Autodesk Inventor part; units mm, degrees
ref_plane "YZ Plane" through (0, 0, 0) normal (1, 0, 0) x (0, 1, 0)
ref_plane "XZ Plane" through (0, 0, 0) normal (0, 1, 0) x (-1, 0, 0)
ref_plane "XY Plane" through (0, 0, 0) normal (0, 0, 1) x (1, 0, 0)
sketch "Sketch1" plane through (0, 0, 0) normal (0, 0, 1) x (1, 0, 0)
  line L0 (-2.75, 1.59) -> (0, 3.18)
  line L1 (0, -3.18) -> (-2.75, -1.59)
  line L2 (-2.75, 1.59) -> (-2.75, -1.59)
  line L3 (2.75, 1.59) -> (0, 3.18)
  line L4 (0, -3.18) -> (2.75, -1.59)
  line L5 (2.75, 1.59) -> (2.75, -1.59)
  point P0 (0, 0)
extrude "Extrusion1" add sketch "Sketch1" along normal blind 6
sketch "Sketch2" plane through (0, 0, 6) normal (0, 0, 1) x (1, 0, 0)
  circle A0 centre (0, 0) radius 1.5
  dimension "d20" = 3
hole "Hole1" at (0, 0, 6) direction (0, 0, -1) diameter 2.459 depth 8.8 tip angle 118
fillet "Fillet1" radius 0.1 6 edges at (0, 3.18, 3) (2.75, 1.59, 3) (-2.75, 1.59, 3) (2.75, -1.59, 3) (0, -3.18, 3) (-2.75, -1.59, 3)
sketch "Sketch4" plane through (0, 0, 0) normal (0, 0, -1) x (-1, 0, 0)
  circle A0 centre (0, 0) radius 1.5
  dimension "d29" = 3
extrude "Extrusion2" add sketch "Sketch4" along normal blind 6.4
thread "Thread1"
fillet "Fillet2" radius 0.2 1 edges at (1.5, 0, -6.4)
properties part number "spacer 3cm" material "Steel, Mild"
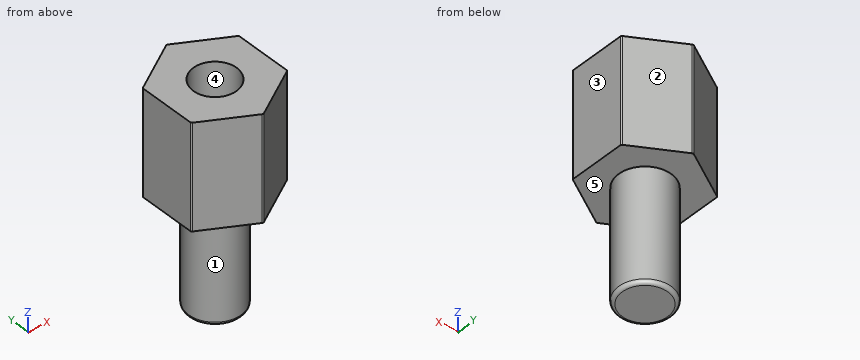
Here's how the part is built. I have some questions about the finished solid (model axes, mm). Face numbers are marked on the shaded views. A direction names the side the tool comes from. Coordinates: 2 decimals unless noted, no trailing zeros. Write each loop counter-clockwise with the first axis right and the second up, starting at its lowest first coordinate (ties: lowest second). Pieces come first, ordered by that corner, then holes. Notation, with made-up numbers: (-10, 37.25) -> (7, 37.25) arc R30 ccw to (7, 68.25) -> close; hole circle Ø11 at (75, -12.75). An arc over 180 degrees is marked (long way). Use a Markdown table: item, result. Add a question column.
(1) For the marked faces 1 and 2, which set-ups out of +Z, -Z, +X, -X, +Y, -Y let a thin tool reach every point of the face, with its end or its side?
(2) We'd pull the mould along X, two halves only. Please class the marked faces 3, 4 and 5: +X half, -X half, draft (parallel to the pull), parting line (faces both ways), or undercut.
(3) If we section it at A-A, the plane z = 3: Write out the boundary of the cut face in (x, y), and give its area (3 significant figures).
(4) If we section it at B-B, the plane y = 0: Write out the boundary of the cut face in (x, z).
(5) If we section it at C-C, the plane z = -3: Write out the boundary of the cut face in (x, y), and give its area (3 significant figures).
(6) I'm going to push flat-ended pins straight in: P1, Ø2, axis at x = 2, z = 4, coming from the +Y side; P2, Ø0.7, axis at x = 0, y = 0, coming from the +Z side. Where does each tip first touch, or does it pass through?
(7) Please list where these lines run through material, in increasing order: line 1 (X direction, y = 0, z = 3); line 2 (Y direction, x = 0, z = 4.6); line 3 (Z direction, x = -1.05, y = -0.25).
Outcome:
| question | item | result |
|---|---|---|
| 1 | face 1 | -Z |
| 1 | face 2 | +Z, -Z, +X, +Y |
| 2 | face 3 | +X half |
| 2 | face 4 | undercut |
| 2 | face 5 | draft |
| 3 | outline | (-2.75, -1.53) arc R0.1 ccw to (-2.7, -1.62) -> (-0.05, -3.15) arc R0.1 ccw to (0.05, -3.15) -> (2.7, -1.62) arc R0.1 ccw to (2.75, -1.53) -> (2.75, 1.53) arc R0.1 ccw to (2.7, 1.62) -> (0.05, 3.15) arc R0.1 ccw to (-0.05, 3.15) -> (-2.7, 1.62) arc R0.1 ccw to (-2.75, 1.53) -> close; hole circle Ø2.46 at (0, 0) |
| 3 | area | 21.5 mm^2 |
| 4 | outline | (-2.75, 0) -> (-1.5, 0) -> (-1.5, -6.2) arc R0.2 ccw to (-1.3, -6.4) -> (1.3, -6.4) arc R0.2 ccw to (1.5, -6.2) -> (1.5, 0) -> (2.75, 0) -> (2.75, 6) -> (1.23, 6) -> (1.23, 0) -> (-1.23, 0) -> (-1.23, 6) -> (-2.75, 6) -> close |
| 5 | outline | circle Ø3 at (0, 0) |
| 5 | area | 7.07 mm^2 |
| 6 | P1 | stops at y = 2.6 |
| 6 | P2 | stops at z = 0 |
| 7 | line 1 | x = -2.75 to -1.23, 1.23 to 2.75 |
| 7 | line 2 | y = -3.16 to -1.23, 1.23 to 3.16 |
| 7 | line 3 | z = -6.4 to 0 |
